Source: CAD feature listing. Evaluate the final solid. Frame: model axes, mm. Face numbers are marked on the shaded views. A direction names the side the tool comes from. Coordinates: 2 decimals unless noted, no trailing zeros. Loops run counter-clockwise (first coordinate to the right, second up) from the corner with the lowest first, then second, coordinate; pieces in that order, holes last. Notation, with made-up numbers: M 0.5,-18 L 53.5,-18 A4 ccw 53.5,-13 Z; hole C -3.5,-34.5 d1. An arc over 180 degrees is marked long. One line per question, with ' | ' between items. Start each with the question number.
1. Access query for the marked faces 1 and 2. Directions: +Z, -Z, +X, -X, +Y, -Y. A direction counts if a zero-diameter tool reaches every point of the face in a straight line with its end or side. Return the directions, or none.
2. Pin query (flat end, axial travel): P1, Ø1.6, axis at x = 3, y = 3, coming from the -Z side; P2, Ø1.2, axis at x = 36, y = 1, coming from the -Z side; P3, Ø2, axis at x = 54, y = 3, coming from the +Z side. Return the tip coordinate at first contact, or that it passes through.
3. Section query A-A, the plane z = -6.9. Output: boundary loops of the cut face in (x, y), and give its area (3 significant figures).
4. Section query D-D, the plane y = 1.6. Output: boundary loops of the cut face in (x, z), and give its area (3 significant figures).
5. Section query B-B, the plane x = 28.5. Output: boundary loops of the cut face in (y, z), and give its area (3 significant figures).
6. Ray query, probe 1 along X at (y, z) = (3.8, -9); probe 2 along X at (y, z) = (4, -8.5); probe 3 along Y at (x, z) = (46, -9.25). Return the intervals inside material, ascending.
7. Section query C-C, the plane x = 10.4. Output: boundary loops of the cut face in (y, z).
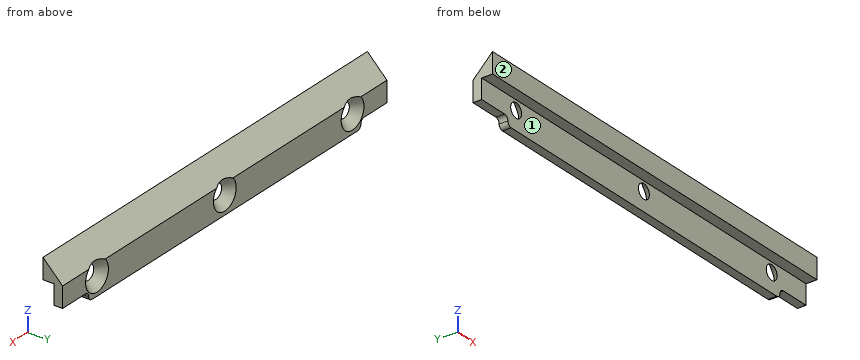
Autodesk Inventor part; units mm, degrees
ref_plane "YZ Plane" through (0, 0, 0) normal (1, 0, 0) x (0, 1, 0)
ref_plane "XZ Plane" through (0, 0, 0) normal (0, 1, 0) x (-1, 0, 0)
ref_plane "XY Plane" through (0, 0, 0) normal (0, 0, 1) x (1, 0, 0)
sketch "Szkic1" plane through (0, 0, 0) normal (1, 0, 0) x (0, 1, 0)
  line L0 (0, 0) -> (4.5, -4.5)
  line L1 (4.5, -4.5) -> (4.5, -11.2)
  line L2 (4.5, -11.2) -> (2.5, -11.2)
  line L3 (2.5, -11.2) -> (2.5, -4.7)
  line L4 (2.5, -4.7) -> (0, -4.7)
  line L5 (0, -4.7) -> (0, 0)
  line L6 (2.5, -4.7) -> (2.5, -2.5) construction
  dimension "d0" = 11.2
  dimension "d1" = 4.5
  dimension "d2" = 45
  dimension "d3" = 2.5
  dimension "d4" = 6.5
extrude "Wyciągnięcie proste1" add sketch "Szkic1" along normal blind 98
sketch "Szkic2" plane through (0, 4.5, -4.5) normal (0, 1, 0) x (1, 0, 0)
  line L0 (0, 6.7) -> (0, 0.2)
  line L1 (0, 6.7) -> (7.9, 6.7)
  line L2 (7.9, 6.7) -> (7.9, 4.7)
  line L3 (7.9, 4.7) -> (0, 4.7)
  line L4 (0, 4.7) -> (0, 6.7)
  line L5 (0, 0.2) -> (98, 0.2) construction
  line L6 (49, 0.2) -> (49, 6.7) construction
  line L7 (0, 6.7) -> (98, 6.7) construction
  line L8 (98, 6.7) -> (90.1, 6.7)
  line L9 (90.1, 6.7) -> (90.1, 4.7)
  line L10 (90.1, 4.7) -> (98, 4.7)
  line L11 (98, 4.7) -> (98, 6.7)
  point P0 (0, -4.5)
  dimension "d7" = 7.9
  dimension "d8" = 2
extrude "Wyciągnięcie proste2" cut sketch "Szkic2" against normal through all
sketch "Szkic3" plane through (0, 4.5, -4.5) normal (0, 1, 0) x (1, 0, 0)
  line L0 (0, -4.5) -> (98, -4.5) construction
  line L1 (49, -4.5) -> (49, 6.7) construction
  line L2 (7.9, 6.7) -> (90.1, 6.7) construction
  line L3 (98, 4.7) -> (98, 0) construction
  point P0 (87.6, 2.4)
  point P1 (49, 2.4)
  point P2 (10.4, 2.4)
  point P3 (98, 0.2)
  dimension "d11" = 10.4
  dimension "d21" = 2.2
hole "Otwór1" at (87.6, 4.5, -6.9) at (49, 4.5, -6.9) at (10.4, 4.5, -6.9) direction (0, -1, 0) diameter 3.2 end through all countersink diameter 6.9 countersink angle 84.225
fillet "Zaokrąglenie1" radius 1 4 edges at (90.1, 3.4707, -9.2) (90.1, 3.5, -11.2) (7.9, 3.4707, -9.2) (7.9, 3.5, -11.2)
properties part number "Plog2" material "Stal"
Taken from the geometry:
1) face 1: -Z, +X, -X, -Y | face 2: +Z, -Z, +X, -X, -Y
2) P1: z = -9.2 | P2: z = -4.7 | P3: z = -2
3) outline: M 0,2.5 L 8.76,2.5 L 6.95,4.5 L 0,4.5 Z; M 12.04,2.5 L 47.36,2.5 L 45.55,4.5 L 13.85,4.5 Z; M 50.64,2.5 L 85.96,2.5 L 84.15,4.5 L 52.45,4.5 Z; M 89.24,2.5 L 98,2.5 L 98,4.5 L 91.05,4.5 Z | area: 165 mm^2
4) outline: M 0,-4.7 L 98,-4.7 L 98,-1.6 L 0,-1.6 Z | area: 304 mm^2
5) outline: M 0,-4.7 L 2.5,-4.7 L 2.5,-11.2 L 4.5,-11.2 L 4.5,-4.5 L 0,0 Z | area: 24.0 mm^2
6) probe 1: 0 to 8.52, 12.28 to 47.12, 50.88 to 85.72, 89.48 to 98 | probe 2: 0 to 7.86, 12.94 to 46.46, 51.54 to 85.06, 90.14 to 98 | probe 3: 2.5 to 4.5
7) outline: M 0,-4.7 L 2.5,-4.7 L 2.5,-5.26 L 3.95,-3.95 L 0,0 Z; M 2.5,-11.2 L 4.5,-11.2 L 4.5,-10.35 L 2.5,-8.54 Z
